```python
from build123d import *

# Parameters (mm, degrees)
SKETCH1_R           = 1.75
BOSS_EXTRUDE1_DEPTH = 50
CUT_EXTRUDE1_DEPTH  = 50
CUT_EXTRUDE2_DEPTH  = 50


with BuildPart() as part:
    # Sketch1 → Boss-Extrude1 (new body)
    with BuildSketch(Plane.XY):
        with BuildLine():
            Line((18.5, -21.5), (-18.5, -21.5))
            ThreePointArc((-18.5, -21.5), (-20.621320344, -20.621320344), (-21.5, -18.5))
            Line((-21.5, -18.5), (-21.5, 18.5))
            ThreePointArc((-21.5, 18.5), (-20.621320344, 20.621320344), (-18.5, 21.5))
            Line((-18.5, 21.5), (18.5, 21.5))
            ThreePointArc((18.5, 21.5), (20.621320344, 20.621320344), (21.5, 18.5))
            Line((21.5, 18.5), (21.5, 14.5))
            ThreePointArc((21.5, 14.5), (20.621320344, 12.378679656), (18.5, 11.5))
            Line((18.5, 11.5), (14.491376746, 11.5))
            ThreePointArc((14.491376746, 11.5), (13.343738663, 11.728190694), (12.370687466, 12.37804878))
            ThreePointArc((12.370687466, 12.37804878), (-17.5, 0), (12.370687466, -12.37804878))
            ThreePointArc((12.370687466, -12.37804878), (13.343738663, -11.728190694), (14.491376746, -11.5))
            Line((14.491376746, -11.5), (18.5, -11.5))
            ThreePointArc((18.5, -11.5), (20.621320344, -12.378679656), (21.5, -14.5))
            Line((21.5, -14.5), (21.5, -18.5))
            ThreePointArc((21.5, -18.5), (20.621320344, -20.621320344), (18.5, -21.5))
        make_face()
        with Locations((-15.5, 15.5)):
            Circle(SKETCH1_R, mode=Mode.SUBTRACT)
        with Locations((-15.5, -15.5)):
            Circle(SKETCH1_R, mode=Mode.SUBTRACT)
        with Locations((15.5, -15.5)):
            Circle(SKETCH1_R, mode=Mode.SUBTRACT)
        with Locations((15.5, 15.5)):
            Circle(SKETCH1_R, mode=Mode.SUBTRACT)
    extrude(amount=BOSS_EXTRUDE1_DEPTH)

    # Sketch2 → Cut-Extrude1 (cut)
    with BuildSketch(Plane(origin=(0, 21.5, 0), x_dir=(1, 0, 0), z_dir=(0, 1, 0))):
        with BuildLine():
            Line((-0.01, -45), (0.01, -45))
            ThreePointArc((0.01, -45), (3.538462838, -43.538462838), (5, -40.01))
            Line((5, -40.01), (5, -9.99))
            ThreePointArc((5, -9.99), (3.538462838, -6.461537162), (0.01, -5))
            Line((0.01, -5), (-0.01, -5))
            ThreePointArc((-0.01, -5), (-3.538462838, -6.461537162), (-5, -9.99))
            Line((-5, -9.99), (-5, -40.01))
            ThreePointArc((-5, -40.01), (-3.538462838, -43.538462838), (-0.01, -45))
        make_face()
    extrude(amount=-CUT_EXTRUDE1_DEPTH, mode=Mode.SUBTRACT)

    # Sketch3 → Cut-Extrude2 (cut)
    with BuildSketch(Plane.ZY.offset(21.5)):
        with BuildLine():
            Line((9.99, -5), (40.01, -5))
            ThreePointArc((40.01, -5), (43.538462838, -3.538462838), (45, -0.01))
            Line((45, -0.01), (45, 0.01))
            ThreePointArc((45, 0.01), (43.538462838, 3.538462838), (40.01, 5))
            Line((40.01, 5), (9.99, 5))
            ThreePointArc((9.99, 5), (6.461537162, 3.538462838), (5, 0.01))
            Line((5, 0.01), (5, -0.01))
            ThreePointArc((5, -0.01), (6.461537162, -3.538462838), (9.99, -5))
        make_face()
    extrude(amount=-CUT_EXTRUDE2_DEPTH, mode=Mode.SUBTRACT)


solid = part.part
```
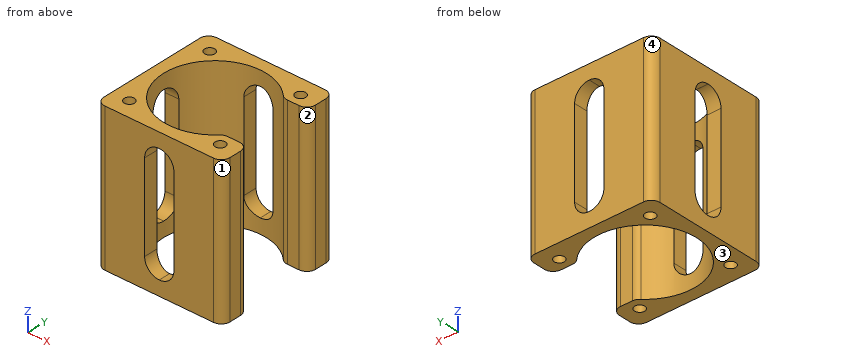
Could you check a few things on this model? Use its own coordinates, in mm. Face numbers are marked on the shaded views. Coordinates: 2 decimals unless noted, no trailing zeros. Loops run counter-clockwise (first coordinate to the right, second up) from the corner with the lowest first, then second, coordinate; pieces in that order, holes last.
1) Thinking about a two-plate mould opening in Y: for the marked faces 1, 2, 3 and 4, which applies, released by +Y, released by -Y, zero draft, split by the parting line, or undercut?
Reported:
face 1: released by -Y
face 2: undercut
face 3: zero draft
face 4: released by +Y
2) Please list where these lines run through material, in increasing order: line 1 along Y through (x, z) = (15.5, 36.5); line 2 along X through (y, z) = (-15, 11); line 3 along X through (y, z) = (-18.5, 32.5).
Reported:
line 1: y = -21.5 to -17.25, -13.75 to -11.5, 11.5 to 13.75, 17.25 to 21.5
line 2: x = -21.5 to -17.18, -13.82 to -9.01, 9.01 to 13.82, 17.18 to 21.5
line 3: x = -21.5 to -5, 5 to 21.5
3) Imagine slicing it at C-C (x = -15.5). List the corners of the cut face in (y, z) for me, and give its area (3 significant figures).
Reported:
outline: (-21.5, 0) - (-17.25, 0) - (-17.25, 50) - (-21.5, 50) - close; (-13.75, 0) - (-8.12, 0) - (-8.12, 50) - (-13.75, 50) - close; (8.12, 0) - (13.75, 0) - (13.75, 50) - (8.12, 50) - close; (17.25, 0) - (21.5, 0) - (21.5, 50) - (17.25, 50) - close
area: 988 mm2
4) Imagine slicing it at B-B (x = -9). List the corners of the cut face in (y, z) for me.
Reported:
outline: (-21.5, 0) - (-15.01, 0) - (-15.01, 50) - (-21.5, 50) - close; (15.01, 0) - (21.5, 0) - (21.5, 50) - (15.01, 50) - close
5) Imagine slicing it at A-A (z = 30). State how many separate pieces and enclosed holes the cut face has, and give its area (3 significant figures).
Reported:
separate pieces: 4
enclosed holes: 4
area: 586 mm2
6) Will these pins go through, and if not, where does the flat tip stop? pin 1 Ø1.5 at (y, z) = (13, 18.5) entering from +X; pin 2 Ø1.4 at (y, z) = (-20, 20.5) entering from -X; pin 3 Ø1.4 at (y, z) = (-19.5, 32.5) entering from +X.
Reported:
pin 1: stops at x = 21.4
pin 2: stops at x = -21.39
pin 3: stops at x = 21.48
